```python
from build123d import *

# Parameters (mm, degrees)
SKETCH1_W                      = 31.877
SKETCH1_H                      = 38.1
BASE_FLANGE1_DEPTH             = 3.175
EDGE_FLANGE1_STRIP_W           = 22.225
EDGE_FLANGE1_STRIP_H           = 3.175
EDGE_FLANGE1_STRIP_CUT_DEPTH   = 38.1
EDGE_FLANGE1_STRIP_2_W         = 22.225
EDGE_FLANGE1_STRIP_2_H         = 3.175
EDGE_FLANGE1_STRIP_CUT_2_DEPTH = 38.1
EDGE_FLANGE1_DEPTH             = 38.1
EDGE_FLANGE1_BEND_DEPTH        = 38.1
CUT_EXTRUDE1_DEPTH             = 95.152162324
CUT_EXTRUDE1_DEPTH_BACK        = 95.152162324
SKETCH12_R                     = 13.335
BREAK_CORNER1_START            = 0.424763322
BREAK_CORNER1_DEPTH            = 31.877


# Read off the part's stored shape, not the designer's step: Break-Corner1
# Sheet-metal steps are written as plain solids
with BuildPart() as part:
    # Sketch1 → Base-Flange1 (new body)
    with BuildSketch(Plane.XY.offset(-38.1)):
        with Locations((16.363263322, 19.05)):
            Rectangle(SKETCH1_W, SKETCH1_H)
    extrude(amount=-BASE_FLANGE1_DEPTH)

    # Edge-Flange1 strip (across the edge) → Edge-Flange1 strip cut (cut)
    with BuildSketch(Plane(origin=(32.301763322, 38.1, -41.275), x_dir=(-1, 0, 0), z_dir=(0, -1, 0))):
        with Locations((-3.175, -1.5875)):
            Rectangle(EDGE_FLANGE1_STRIP_W, EDGE_FLANGE1_STRIP_H)
    extrude(amount=EDGE_FLANGE1_STRIP_CUT_DEPTH, mode=Mode.SUBTRACT)

    # Edge-Flange1 strip 2 (across the edge) → Edge-Flange1 strip cut 2 (cut)
    with BuildSketch(Plane(origin=(0.424763322, 0, -41.275), x_dir=(1, 0, 0), z_dir=(0, 1, 0))):
        with Locations((-3.175, -1.5875)):
            Rectangle(EDGE_FLANGE1_STRIP_2_W, EDGE_FLANGE1_STRIP_2_H)
    extrude(amount=EDGE_FLANGE1_STRIP_CUT_2_DEPTH, mode=Mode.SUBTRACT)

    # Edge-Flange1 section (across the edge) → Edge-Flange1 (add)
    with BuildSketch(Plane(origin=(32.301763322, 38.1, -41.275), x_dir=(-1, 0, 0), z_dir=(0, -1, 0))):
        with BuildLine():
            Line((0, 4.7625), (0, 38.534872551))
            Line((0, 38.534872551), (3.175, 38.534872551))
            Line((3.175, 38.534872551), (3.175, 4.7625))
            ThreePointArc((3.175, 4.7625), (4.569903955, 1.394903955), (7.9375, 0))
            Line((7.9375, 0), (7.9375, -3.175))
            ThreePointArc((7.9375, -3.175), (2.324839924, -0.850160076), (0, 4.7625))
        make_face()
    extrude(amount=EDGE_FLANGE1_DEPTH)

    # Edge-Flange1 section 2 (across the edge) → Edge-Flange1 bend (add)
    with BuildSketch(Plane(origin=(0.424763322, 0, -41.275), x_dir=(1, 0, 0), z_dir=(0, 1, 0))):
        with BuildLine():
            Line((0, 4.7625), (0, 38.534872551))
            Line((0, 38.534872551), (3.175, 38.534872551))
            Line((3.175, 38.534872551), (3.175, 4.7625))
            ThreePointArc((3.175, 4.7625), (4.569903955, 1.394903955), (7.9375, 0))
            Line((7.9375, 0), (7.9375, -3.175))
            ThreePointArc((7.9375, -3.175), (2.324839924, -0.850160076), (0, 4.7625))
        make_face()
    extrude(amount=EDGE_FLANGE1_BEND_DEPTH)

    # Sketch12 → Cut-Extrude1 (cut, two sides: drawn at the far end of the back side and taken through both)
    with BuildSketch(Plane(origin=(0, 0, 0), x_dir=(0, 0, -1), z_dir=(1, 0, 0)).offset(-CUT_EXTRUDE1_DEPTH_BACK)):
        with Locations((79.809872551, 0)):
            Circle(SKETCH12_R)
    extrude(amount=CUT_EXTRUDE1_DEPTH + CUT_EXTRUDE1_DEPTH_BACK, mode=Mode.SUBTRACT)

    # Break-Corner1 outline → Break-Corner1 (cut)
    with BuildSketch(Plane.YZ.offset(BREAK_CORNER1_START)):
        with BuildLine():
            Line((13.335, -79.809872551), (18.632678954, -79.809872551))
            ThreePointArc((18.632678954, -79.809872551), (14.937057089, -78.623677256), (12.622137356, -75.508259648))
            ThreePointArc((12.622137356, -75.508259648), (13.15557727, -77.629732262), (13.335, -79.809872551))
        make_face()
        with BuildLine():
            ThreePointArc((38.1, -73.459872551), (36.24012806, -77.950000612), (31.75, -79.809872551))
            Line((31.75, -79.809872551), (38.1, -79.809872551))
            Line((38.1, -79.809872551), (38.1, -73.459872551))
        make_face()
        with BuildLine():
            ThreePointArc((0, -66.474872551), (2.180140289, -66.654295281), (4.301612903, -67.187735195))
            ThreePointArc((4.301612903, -67.187735195), (1.186195295, -64.872815462), (0, -61.177193597))
            Line((0, -61.177193597), (0, -66.474872551))
        make_face()
    extrude(amount=BREAK_CORNER1_DEPTH, mode=Mode.SUBTRACT)


solid = part.part
```
Work out the finished part from the listing and answer in its coordinate system (mm). A direction names the side the tool comes from. Give positions to 0.01 mm unless a question says otherwise; leave off trailing zeros. Order: outer loops, then holes, each group sorted by start corner. A loop starts at its lowest first (then second) coordinate and runs counter-clockwise, first axis right, second up.
1. Section C-C, the plane x = 14 is taken. Determine the outline of the cut face in (y, z) (3 decimals), and give its area (3 significant figures).
Result sheet:
outline: (0, -41.275) - (38.1, -41.275) - (38.1, -38.1) - (0, -38.1) - close
area: 121 mm2
2. The mould has two halves that part along X. Classify faces 1 (the cylindrical face through (30.69, 36.29, -77.9)), 2 (the flat face through (0.425, 19, -63)), 3 (the flat face through (16, 19, -41.275)): released by +X, released by -X, zero draft, split by the parting line, or undercut.
Result sheet:
face 1: zero draft
face 2: released by -X
face 3: undercut
3. Each of these flat-tipped pins is pushed along its axis until it touches: P1, Ø6, axis at x = 19, y = 25, coming from the -Z side (3 decimals); P2, Ø8, axis at x = 11.5, z = -71.5, coming from the -Y side; P3, Ø5, axis at x = 28.5, z = -57, coming from the +Y side. Where does it stop, or does it pass through?
Result sheet:
P1: stops at z = -41.275
P2: passes through
P3: stops at y = 38.1
4. Section A-A, the plane z = -54.5 is taken. Determine the outline of the cut face in (x, y), and give its area (3 significant figures).
Result sheet:
outline: (0.42, 0) - (3.6, 0) - (3.6, 38.1) - (0.42, 38.1) - close; (29.13, 0) - (32.3, 0) - (32.3, 38.1) - (29.13, 38.1) - close
area: 242 mm2
5. Straight lines are drawn through the part: L1, parallel to X at y = 3, z = -62; L2, parallel to Z at x = 22, y = 36 (3 decimals); L3, parallel to Z at x = 6, y = 13. For each, find the intervals that lie inside material, in ascending order.
Result sheet:
L1: x = 0.42 to 3.6, 29.13 to 32.3
L2: z = -41.275 to -38.1
L3: z = -41.9 to -38.46
6. For faces 4 (the cylindrical face through (4.958, 18.783, -42.707)), 5 (the flat face through (2, 25, -79.81)), determine the directions among +Z, -Z, +X, -X, +Y, -Y from which every point of the face is accessible in a straight line to the end or side of a thin tool.
Result sheet:
face 4: -Z, +Y, -Y
face 5: -Z, +X, -X, +Y, -Y
7. Section B-B, the plane y = 12 is taken. Determine the outline of the cut face in (x, z) (1 decimal).
Result sheet:
outline: (0.4, -74) - (3.6, -74) - (3.6, -46) arc R4.8 cw to (8.4, -41.3) - (24.4, -41.3) arc R4.8 cw to (29.1, -46) - (29.1, -74) - (32.3, -74) - (32.3, -46) arc R7.9 ccw to (24.4, -38.1) - (8.4, -38.1) arc R7.9 ccw to (0.4, -46) - close
8. Section D-D, the plane z = -62 is taken. Determine the outline of the cut face in (x, y), and give its area (3 significant figures).
Result sheet:
outline: (0.42, 0.05) - (3.6, 0.05) - (3.6, 38.1) - (0.42, 38.1) - close; (29.13, 0.05) - (32.3, 0.05) - (32.3, 38.1) - (29.13, 38.1) - close
area: 242 mm2
